```python
from build123d import *

# Parameters (mm, degrees)
CHAMFER1_SIZE                  = 1.5875
CHAMFER2_SIZE                  = 1.27
CUT_EXTRUDE4_REACH             = 73.102
SKETCH2_R                      = 3.96875
SKETCH2_R_2                    = 1.5875
SKETCH2_R_3                    = 0.79375
CUT_EXTRUDE4_DIRECTION_2_REACH = 73.102
CUT_EXTRUDE5_REACH             = 73.102
CUT_EXTRUDE5_END_RADIUS        = 6.35
SKETCH3_R                      = 3.175
CUT_EXTRUDE7_START             = -50.8
CUT_EXTRUDE7_DEPTH             = 50.8


with BuildPart() as part:
    # Sketch1 → Revolve1 (revolve)
    with BuildSketch(Plane(origin=(0, 0, 0), x_dir=(0, 0, -1), z_dir=(1, 0, 0))):
        Polygon((0, 41.275), (0, 66.675), (-7.9375, 66.675), (-7.9375, 60.325), (-6.35, 60.325), (-6.35, 47.625), (-7.9375, 47.625), (-7.9375, 41.275), (-3.96875, 41.275), align=None)
        Polygon((0, 28.575), (0, 41.275), (-3.96875, 41.275), (-4.7625, 28.575), align=None)
        Polygon((0, 15.875), (0, 28.575), (-4.7625, 28.575), (-7.9375, 28.575), (-7.9375, 15.875), (-7.493, 15.875), (-4.7625, 15.875), align=None)
        with BuildLine():
            Line((0, 11.165242708), (0, 15.875))
            Line((0, 15.875), (-4.7625, 15.875))
            add(Edge.make_bspline(
                [(-4.7625, 15.875), (-4.599205469, 15.673771419), (-4.529160375, 15.219340562), (-4.601951333, 14.659365635), (-4.863719246, 13.209599289), (-5.693032567, 11.944502432), (-6.477, 11.165242708)],
                knots=[0, 0, 0, 0, 0.134423487, 0.277975298, 0.329406914, 1, 1, 1, 1], degree=3))
            Line((-6.477, 11.165242708), (0, 11.165242708))
        make_face()
        with BuildLine():
            Line((0, 6.35), (0, 11.165242708))
            Line((0, 11.165242708), (-6.477, 11.165242708))
            Line((-6.477, 11.165242708), (-7.493, 11.165242708))
            ThreePointArc((-7.493, 11.165242708), (-9.525, 9.133242708), (-7.493, 7.101242708))
            ThreePointArc((-7.493, 7.101242708), (-7.21765082, 6.725621354), (-7.493, 6.35))
            Line((-7.493, 6.35), (0, 6.35))
        make_face()
        Polygon((0, 4.7625), (0, 6.35), (-7.493, 6.35), (-9.525, 6.35), (-9.525, 4.7625), align=None)
        Polygon((0, 0), (0, 4.7625), (-9.525, 4.7625), (-17.4625, 4.7625), (-17.4625, 0), align=None)
    revolve(axis=Axis((0, 73.617342774, 0), (0, -1, 0)))

    # Chamfer1
    chamfer1_edges = [part.edges().sort_by_distance(p)[0] for p in [
        (0, 4.7625, -17.4625),
    ]]
    chamfer(chamfer1_edges, length=CHAMFER1_SIZE)

    # Chamfer2
    chamfer2_edges = [part.edges().sort_by_distance(p)[0] for p in [
        (0, 15.875, -7.9375),
        (0, 28.575, -7.9375),
    ]]
    chamfer(chamfer2_edges, length=CHAMFER2_SIZE)

    # Sketch2 → Cut-Extrude4 (cut, up to next)
    with BuildSketch(Plane(origin=(0, 0, 0), x_dir=(0, 0, -1), z_dir=(1, 0, 0)), mode=Mode.PRIVATE) as cut_extrude4_sk1:
        with Locations(Location((0, 22.225, 0), (0, 0, 180))):
            Circle(SKETCH2_R)
    cut_extrude4_tool1 = extrude(cut_extrude4_sk1.sketch, amount=-CUT_EXTRUDE4_REACH, mode=Mode.PRIVATE) & part.part
    # Sketch2 → Cut-Extrude4 (cut, up to next)
    with BuildSketch(Plane(origin=(0, 0, 0), x_dir=(0, 0, -1), z_dir=(1, 0, 0)), mode=Mode.PRIVATE) as cut_extrude4_sk2:
        with Locations(Location((0, 53.975, 0), (0, 0, 180))):
            Circle(SKETCH2_R_2)
    cut_extrude4_tool2 = extrude(cut_extrude4_sk2.sketch, amount=-CUT_EXTRUDE4_REACH, mode=Mode.PRIVATE) & part.part
    # Sketch2 → Cut-Extrude4 (cut, up to next)
    with BuildSketch(Plane(origin=(0, 0, 0), x_dir=(0, 0, -1), z_dir=(1, 0, 0)), mode=Mode.PRIVATE) as cut_extrude4_sk3:
        with Locations(Location((-1.864995, 63.307976, 0), (0, 0, 180))):
            Circle(SKETCH2_R_3)
    cut_extrude4_tool3 = extrude(cut_extrude4_sk3.sketch, amount=-CUT_EXTRUDE4_REACH, mode=Mode.PRIVATE) & part.part
    # Sketch2 → Cut-Extrude4 (cut, up to next)
    with BuildSketch(Plane(origin=(0, 0, 0), x_dir=(0, 0, -1), z_dir=(1, 0, 0)), mode=Mode.PRIVATE) as cut_extrude4_sk4:
        with Locations(Location((1.864995, 63.307976, 0), (0, 0, 180))):
            Circle(SKETCH2_R_3)
    cut_extrude4_tool4 = extrude(cut_extrude4_sk4.sketch, amount=-CUT_EXTRUDE4_REACH, mode=Mode.PRIVATE) & part.part
    add(cut_extrude4_tool1.solids().sort_by_distance((0, 22.225, 0))[0], mode=Mode.SUBTRACT)
    add(cut_extrude4_tool2.solids().sort_by_distance((0, 53.975, 0))[0], mode=Mode.SUBTRACT)
    add(cut_extrude4_tool3.solids().sort_by_distance((0, 63.307976, 1.864995))[0], mode=Mode.SUBTRACT)
    add(cut_extrude4_tool4.solids().sort_by_distance((0, 63.307976, -1.864995))[0], mode=Mode.SUBTRACT)

    # Sketch2 → Cut-Extrude4 direction 2 (cut, up to next)
    with BuildSketch(Plane(origin=(0, 0, 0), x_dir=(0, 0, -1), z_dir=(1, 0, 0)), mode=Mode.PRIVATE) as cut_extrude4_direction_2_sk1:
        with Locations(Location((0, 22.225, 0), (0, 0, 180))):
            Circle(SKETCH2_R)
    cut_extrude4_direction_2_tool1 = extrude(cut_extrude4_direction_2_sk1.sketch, amount=CUT_EXTRUDE4_DIRECTION_2_REACH, mode=Mode.PRIVATE) & part.part
    # Sketch2 → Cut-Extrude4 direction 2 (cut, up to next)
    with BuildSketch(Plane(origin=(0, 0, 0), x_dir=(0, 0, -1), z_dir=(1, 0, 0)), mode=Mode.PRIVATE) as cut_extrude4_direction_2_sk2:
        with Locations(Location((0, 53.975, 0), (0, 0, 180))):
            Circle(SKETCH2_R_2)
    cut_extrude4_direction_2_tool2 = extrude(cut_extrude4_direction_2_sk2.sketch, amount=CUT_EXTRUDE4_DIRECTION_2_REACH, mode=Mode.PRIVATE) & part.part
    # Sketch2 → Cut-Extrude4 direction 2 (cut, up to next)
    with BuildSketch(Plane(origin=(0, 0, 0), x_dir=(0, 0, -1), z_dir=(1, 0, 0)), mode=Mode.PRIVATE) as cut_extrude4_direction_2_sk3:
        with Locations(Location((-1.864995, 63.307976, 0), (0, 0, 180))):
            Circle(SKETCH2_R_3)
    cut_extrude4_direction_2_tool3 = extrude(cut_extrude4_direction_2_sk3.sketch, amount=CUT_EXTRUDE4_DIRECTION_2_REACH, mode=Mode.PRIVATE) & part.part
    # Sketch2 → Cut-Extrude4 direction 2 (cut, up to next)
    with BuildSketch(Plane(origin=(0, 0, 0), x_dir=(0, 0, -1), z_dir=(1, 0, 0)), mode=Mode.PRIVATE) as cut_extrude4_direction_2_sk4:
        with Locations(Location((1.864995, 63.307976, 0), (0, 0, 180))):
            Circle(SKETCH2_R_3)
    cut_extrude4_direction_2_tool4 = extrude(cut_extrude4_direction_2_sk4.sketch, amount=CUT_EXTRUDE4_DIRECTION_2_REACH, mode=Mode.PRIVATE) & part.part
    add(cut_extrude4_direction_2_tool1.solids().sort_by_distance((0, 22.225, 0))[0], mode=Mode.SUBTRACT)
    add(cut_extrude4_direction_2_tool2.solids().sort_by_distance((0, 53.975, 0))[0], mode=Mode.SUBTRACT)
    add(cut_extrude4_direction_2_tool3.solids().sort_by_distance((0, 63.307976, 1.864995))[0], mode=Mode.SUBTRACT)
    add(cut_extrude4_direction_2_tool4.solids().sort_by_distance((0, 63.307976, -1.864995))[0], mode=Mode.SUBTRACT)

    # Cut-Extrude5: up to this cylinder (the profile starts inside it)
    cut_extrude5_end = Plane(origin=(0, 53.975, 0), z_dir=(0, 1, 0)) * Cylinder(CUT_EXTRUDE5_END_RADIUS, 159.904, mode=Mode.PRIVATE)
    # Sketch3 → Cut-Extrude5 (cut, up to the surface)
    with BuildSketch(Plane(origin=(0, 0, 0), x_dir=(0, 0, -1), z_dir=(1, 0, 0)), mode=Mode.PRIVATE) as cut_extrude5_sk1:
        with Locations((0, 53.975)):
            Circle(SKETCH3_R)
    cut_extrude5_tool1 = extrude(cut_extrude5_sk1.sketch, amount=-CUT_EXTRUDE5_REACH, mode=Mode.PRIVATE) & cut_extrude5_end
    add(cut_extrude5_tool1.solids().sort_by_distance((0, 53.975, 0))[0], mode=Mode.SUBTRACT)

    # Sketch5 → Cut-Extrude7 (cut)
    with BuildSketch(Plane(origin=(0, 66.675, 0), x_dir=(1, 0, 0), z_dir=(0, 1, 0)).offset(CUT_EXTRUDE7_START)):
        with BuildLine():
            Line((4.7625, 10.702126501), (4.7625, 6.35))
            ThreePointArc((4.7625, 6.35), (7.099515829, 3.549757914), (7.9375, 0))
            Line((7.9375, 0), (7.9375, 10.702126501))
            Line((7.9375, 10.702126501), (4.7625, 10.702126501))
        make_face()
        with BuildLine():
            ThreePointArc((7.9375, 0), (7.099515829, 3.549757914), (4.7625, 6.35))
            Line((4.7625, 6.35), (4.7625, -6.35))
            ThreePointArc((4.7625, -6.35), (7.099515829, -3.549757914), (7.9375, 0))
        make_face()
        with BuildLine():
            ThreePointArc((7.9375, 0), (7.099515829, -3.549757914), (4.7625, -6.35))
            Line((4.7625, -6.35), (4.7625, -10.274895902))
            Line((4.7625, -10.274895902), (7.9375, -10.274895902))
            Line((7.9375, -10.274895902), (7.9375, 0))
        make_face()
    extrude(amount=CUT_EXTRUDE7_DEPTH, mode=Mode.SUBTRACT)


solid = part.part
```
Check sheet for the modelled part. Datum: model origin and axes. Units: mm. A direction names the side the tool comes from. Coordinates: 2 decimals unless noted, no trailing zeros. Write each question's results on one line, items separated by ' | '. Start each with the question number.
1. Access from +Z, -Z, +X, -X, +Y, -Y to the whole of each face (thin tool, end or side, straight path). Record for faces 4 (the face through (-3.131, 52.759, -2.933)), 5 (the face through (-6.87, 28.37, 0.23)), 6 (the face through (5.796, 5.545, -7.559)), 7 (the face through (4.762, 19, -3)).
2. Material ranges on probe 1 along Y at (x, z) = (-2.5, 0) (3 decimals); probe 2 along Y at (x, z) = (3.5, 0) (1 decimal); probe 3 along Y at (x, z) = (7, 10), recorded low to high.
3. Go/stop test with flat-tipped pins: P1, Ø4, axis at x = -1.5, y = 29, coming from the -Z side; P2, Ø5, axis at y = 13, z = 0, coming from the +X side; P3, Ø6, axis at x = -11, z = -3, coming from the +Y side; P4, Ø5, axis at x = -12, z = -9, coming from the -Y side. Record where each tip stops, or that it passes through.
4. Mould release check, pull along Y, two halves, no side actions. Record for faces 1 (the face through (-7.934, 44.406, 0.246)), 2 (the face through (-6.3, 47.625, 1.8)), 3 (the face through (-2, 66.675, 0)): +Y half, -Y half, draft (parallel to the pull), parting line (faces both ways), or undercut.
Checks:
1) face 4: -X | face 5: none | face 6: +Y | face 7: +Z, -Z, +X, +Y
2) probe 1: y = 0 to 18.256, 26.194 to 50.8, 57.15 to 66.675 | probe 2: y = 0 to 18.3, 26.2 to 52.4, 55.6 to 66.7 | probe 3: y = 0 to 4.76
3) P1: stops at z = -7.93 | P2: stops at x = 9 | P3: stops at y = 10.95 | P4: stops at y = 0
4) face 1: draft | face 2: undercut | face 3: +Y half
